```python
from build123d import *

# Parameters (mm, degrees)
F0_R     = 10
F1_DEPTH = 25


# Not quite as in the source:
# - the program builds the solid bodies; features that only make, move or delete a surface that nothing else refers to are left out


with BuildPart() as f1:
    # F0 (on Front) → F1 (new body)
    with BuildSketch(Plane.XZ):
        with BuildLine():
            ThreePointArc((-20, -21.8138062528), (-30.7082507277, -39.2518025849), (-50, -46.0766659346))
            Line((-50, -46.0766659346), (50, -46.0766659346))
            ThreePointArc((50, -46.0766659346), (30.7082507277, -39.2518025849), (20, -21.8138062528))
            Line((20, -21.8138062528), (20, 8.1861937472))
            Line((20, 8.1861937472), (50, 8.1861937472))
            Line((50, 8.1861937472), (50, 41.2879567593))
            Line((50, 41.2879567593), (-50, 41.2879567593))
            Line((-50, 41.2879567593), (-50, 8.1861937472))
            Line((-50, 8.1861937472), (-20, 8.1861937472))
            Line((-20, 8.1861937472), (-20, -21.8138062528))
        make_face()
        with Locations((-20, 26.2879567593)):
            Circle(F0_R, mode=Mode.SUBTRACT)
        with Locations((20, 26.2879567593)):
            Circle(F0_R, mode=Mode.SUBTRACT)
    extrude(amount=F1_DEPTH)


solid = f1.part
```
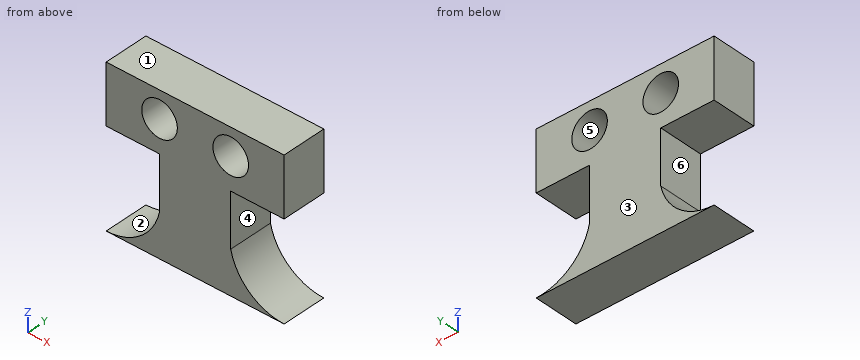
Verification items for the finished model (mm, model axes). Face numbers are marked on the shaded views. A direction names the side the tool comes from. Round coordinates to 2 decimals unless told otherwise and drop trailing zeros. Loops run counter-clockwise (first coordinate to the right, second up) from the corner with the lowest first, then second, coordinate; pieces in that order, holes last. Notation, with made-up numbers: (9, 51) -> (39, 51) arc R7 cw to (39, 58) -> close; hole circle Ø3 at (5, 46). An arc over 180 degrees is marked (long way). Answer as a JSON object with one key per item and string values.
Q1. Access from +Z, -Z, +X, -X, +Y, -Y to the whole of each face (thin tool, end or side, straight path). Record for the marked faces 4, 5 and 6.
Data:
{"face 4": "+X, +Y, -Y", "face 5": "+Y, -Y", "face 6": "-X, +Y, -Y"}
Q2. Section check C-C (x = 39.5). Record the boundary of the cut face in (y, z).
Data:
{"outline": "(-25, -46.08) -> (0, -46.08) -> (0, -44.22) -> (-25, -44.22) -> close; (-25, 8.19) -> (0, 8.19) -> (0, 41.29) -> (-25, 41.29) -> close"}
Q3. Go/stop test with flat-tipped pins: P1, Ø6, axis at y = -22, z = -34, coming from the -X side; P2, Ø2, axis at y = -11, z = -20.5, coming from the -X side; P3, Ø2, axis at x = -25.5, z = -34, coming from the +Y side; P4, Ø12.5, axis at y = -17, z = -3, coming from the +X side. Record where each tip stops, or that it passes through.
Data:
{"P1": "stops at x = -28.22", "P2": "stops at x = -20", "P3": "stops at y = 0", "P4": "stops at x = 20"}
Q4. Section check B-B (y = -19.75). Record the boundary of the cut face in (x, z), then the cut area to 3 significant figures.
Data:
{"outline": "(-50, -46.08) -> (50, -46.08) arc R30.68 cw to (20, -21.81) -> (20, 8.19) -> (50, 8.19) -> (50, 41.29) -> (-50, 41.29) -> (-50, 8.19) -> (-20, 8.19) -> (-20, -21.81) arc R30.68 cw to start; hole circle Ø20 at (-20, 26.29); hole circle Ø20 at (20, 26.29)", "area": "5,220 mm2"}
Q5. Draft check along Z on the marked faces 1, 2 and 3. Enter one of: pulls with the +Z half, pulls with the -Z half, needs draft (parallel to the pull), parting line crosses it, or undercut.
Data:
{"face 1": "pulls with the +Z half", "face 2": "undercut", "face 3": "needs draft"}
Q6. Section check D-D (z = -33.5). Record the boundary of the cut face in (x, y), then the cut area to 3 significant figures.
Data:
{"outline": "(-25.23, -25) -> (25.23, -25) -> (25.23, 0) -> (-25.23, 0) -> close", "area": "1,260 mm2"}
Q7. Section check A-A (x = 14). Record the boundary of the cut face in (y, z).
Data:
{"outline": "(-25, -46.08) -> (0, -46.08) -> (0, 18.29) -> (-25, 18.29) -> close; (-25, 34.29) -> (0, 34.29) -> (0, 41.29) -> (-25, 41.29) -> close"}
Q8. Scan lines: line 1 (X direction, y = -23.75, z = 29); line 2 (X direction, y = -10.25, z = 19); line 3 (Z direction, x = -29, y = -9.5). Record each from-to range of solid material in increasing order. Write a range as from..to.
Data:
{"line 1": "x = -50..-29.63, -10.37..10.37, 29.63..50", "line 2": "x = -50..-26.85, -13.15..13.15, 26.85..50", "line 3": "z = -46.08..-37.76, 8.19..21.93, 30.65..41.29"}
